Verification items for the finished model (mm, model axes). Round coordinates to 2 decimals unless told otherwise and drop trailing zeros. Loops run counter-clockwise (first coordinate to the right, second up) from the corner with the lowest first, then second, coordinate; pieces in that order, holes last. Notation, with made-up numbers: (77.5, 38) -> (113.5, 38) arc R13 cw to (113.5, 62) -> close; hole circle Ø2 at (-18.5, 22.5). An arc over 180 degrees is marked (long way). Write item = value, one per line.
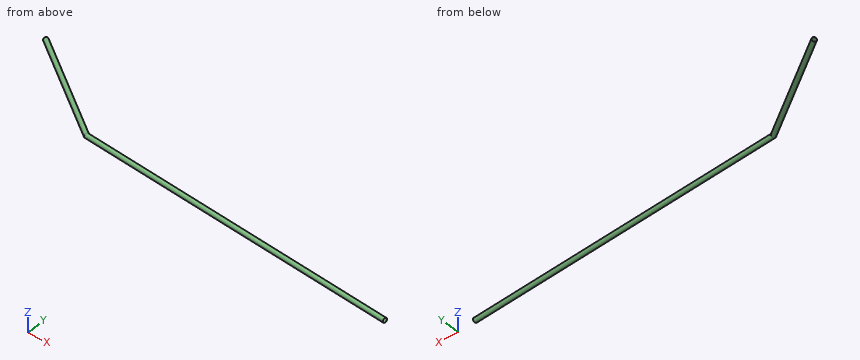
```python
from build123d import *

# Parameters (mm, degrees)
SKETCH3_R   = 2.6
SKETCH3_R_2 = 2.5


with BuildPart() as part:
    # Sweep-Thin1: sweep along a path in Sketch2
    with BuildLine(Plane.XY) as sweep_thin1_path:
        Line((0, 0), (380, 33.24569214))
        Line((380, 33.24569214), (500, 117.270596725))
    # Sketch3 → Sweep-Thin1 (sweep)
    with BuildSketch(Plane(origin=(0, 0, 0), x_dir=(0, 0, -1), z_dir=(0.996194698, 0.087155743, 0))):
        Circle(SKETCH3_R)
        Circle(SKETCH3_R_2, mode=Mode.SUBTRACT)
    sweep(path=sweep_thin1_path.line, transition=Transition.RIGHT)


with BuildPart() as body_2:
    # Mirror1: mirrored copy
    add(part.part.mirror(Plane(origin=(0, 0, 0), x_dir=(0, 0, 1), z_dir=(1, 0, 0))))


solid = body_2.part
```
(1) Go/stop test with flat-tipped pins: pin 1 Ø1.5 at (x, z) = (-203, 1) entering from +Y; pin 2 Ø1 at (x, z) = (-188, -0.5) entering from +Y; pin 3 Ø2 at (x, z) = (-178, 0.5) entering from +Y. Record where each tip stops, or that it passes through.
Filled sheet:
pin_1 = 20.38
pin_2 = 19.09
pin_3 = 18.26
(2) Material ranges on probe 1 along X at (y, z) = (86, 0); probe 2 along X at (y, z) = (96, -1.8); probe 3 along Y at (x, z) = (-175, 2.25), recorded low to high. Write a range as from..to.
Filled sheet:
probe_1 = -459.87..-459.7, -450.98..-450.81
probe_2 = -472.89..-472.65, -466.6..-466.35
probe_3 = 14..14.22, 16.4..16.62
(3) Sectioned sample at A-A, the plane z = 1.15. Record the cut outline in (x, y).
Filled sheet:
outline = (-501.34, 115.36) -> (-380.83, 30.98) -> (-0.2, -2.32) -> (-0.19, -2.21) -> (-380.79, 31.09) -> (-501.27, 115.45) -> close; (-498.73, 119.09) -> (-379.21, 35.41) -> (0.19, 2.21) -> (0.2, 2.32) -> (-379.17, 35.51) -> (-498.66, 119.18) -> close
